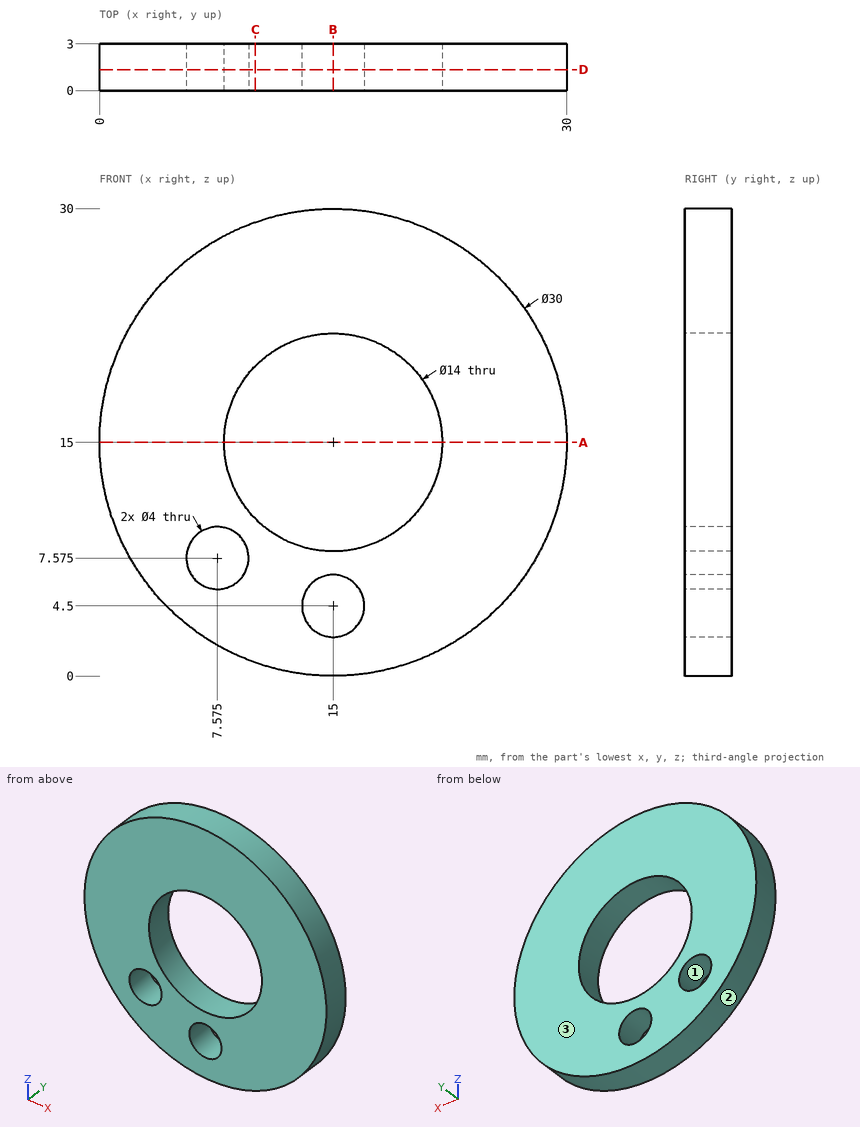
Answer from the drawing. Dimensions are ordinates in mm from the lowest x, y and z of the part. Give positions to 0.01 mm unless a question says otherwise; leave off trailing zeros. Loops run counter-clockwise (first coordinate to the right, second up) from the corner with the lowest first, then second, coordinate; pieces in that order, holes last.
Item 1: A cutting plane is placed at A-A (z = 15). Give the vertices of the cut face in (x, y), then the cut area to 3 significant figures.
Derived:
outline: (0, 0) - (8, 0) - (8, 3) - (0, 3) - close; (22, 0) - (30, 0) - (30, 3) - (22, 3) - close
area: 48.0 mm2
Item 2: Each of these flat-tipped pins is pushed along its axis until it touches: pin 1 Ø2.5 at (x, z) = (15, 4.5) entering from +Y; pin 2 Ø1.5 at (x, y) = (20, 0.5) entering from +Z (1 decimal); pin 3 Ø1.5 at (x, y) = (8.5, 0.5) entering from -Z (1 decimal). Where does it stop, or does it pass through?
Derived:
pin 1: passes through
pin 2: stops at z = 29.4
pin 3: stops at z = 1.1
Item 3: A cutting plane is placed at C-C (x = 10). Give the vertices of the cut face in (y, z).
Derived:
outline: (0, 0.86) - (3, 0.86) - (3, 10.1) - (0, 10.1) - close; (0, 19.9) - (3, 19.9) - (3, 29.14) - (0, 29.14) - close
Item 4: A cutting plane is placed at B-B (x = 15). Give the vertices of the cut face in (y, z).
Derived:
outline: (0, 0) - (3, 0) - (3, 2.5) - (0, 2.5) - close; (0, 6.5) - (3, 6.5) - (3, 8) - (0, 8) - close; (0, 22) - (3, 22) - (3, 30) - (0, 30) - close
Item 5: A cutting plane is placed at D-D (y = 1.35). Give the vertices of the cut face in (x, z) (1 decimal), then the cut area to 3 significant figures.
Derived:
outline: circle Ø30 at (15, 15); hole circle Ø4 at (7.6, 7.6); hole circle Ø14 at (15, 15); hole circle Ø4 at (15, 4.5)
area: 528 mm2
Item 6: Determine the mould class of the marked faces 1, 2 and 3 for opening direction X: +X half, -X half, draft (parallel to the pull), parting line (faces both ways), or undercut.
Derived:
face 1: undercut
face 2: parting line
face 3: draft
Item 7: Find the intervals of material crossed by line 1 along Z through (x, y) = (15, 2.1); line 2 along Z through (x, y) = (12, 2.25) (1 decimal); line 3 along X through (y, z) = (2.3, 14.5), in increasing order.
Derived:
line 1: z = 0 to 2.5, 6.5 to 8, 22 to 30
line 2: z = 0.3 to 8.7, 21.3 to 29.7
line 3: x = 0.01 to 8.02, 21.98 to 29.99
